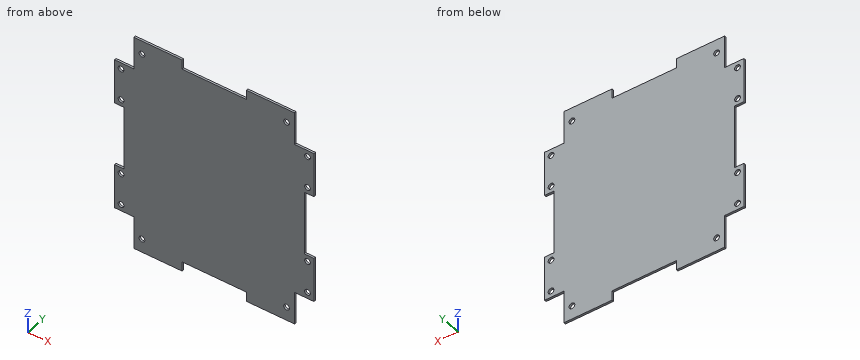
from build123d import *

# Parameters (mm, degrees)
SKETCH1_R           = 2.286
BOSS_EXTRUDE1_DEPTH = 1.5875
SKETCH2_R           = 2.286
CUT_EXTRUDE1_DEPTH  = 2.5875


with BuildPart() as part:
    # Sketch1 → Boss-Extrude1 (new body)
    with BuildSketch(Plane(origin=(0, 0, 0), x_dir=(1, 0, 0), z_dir=(0, 1, 0))):
        Polygon((-25.4, 86.995), (-63.43142, 86.995), (-63.43142, 60.96), (-78.74, 60.96), (-78.74, 25.4), (-71.12, 25.4), (-71.12, -25.4), (-78.74, -25.4), (-78.74, -60.96), (-63.43142, -60.96), (-63.43142, -86.995), (-25.4, -86.995), (-25.4, -79.375), (25.4, -79.375), (25.4, -86.995), (63.43142, -86.995), (63.43142, -60.96), (78.74, -60.96), (78.74, -25.4), (71.12, -25.4), (71.12, 25.4), (78.74, 25.4), (78.74, 60.96), (63.43142, 60.96), (63.43142, 86.995), (25.4, 86.995), (25.4, 79.375), (-25.4, 79.375), align=None)
        with Locations((-57.15, 76.2)):
            Circle(SKETCH1_R, mode=Mode.SUBTRACT)
        with Locations((57.15, 76.2)):
            Circle(SKETCH1_R, mode=Mode.SUBTRACT)
        with Locations((57.15, -76.2)):
            Circle(SKETCH1_R, mode=Mode.SUBTRACT)
        with Locations((-57.15, -76.2)):
            Circle(SKETCH1_R, mode=Mode.SUBTRACT)
    extrude(amount=BOSS_EXTRUDE1_DEPTH)

    # Sketch2 → Cut-Extrude1 (cut, through all)
    with BuildSketch(Plane(origin=(0, 1.5875, 0), x_dir=(1, 0, 0), z_dir=(0, 1, 0))):
        with Locations((-73.66, -30.48)):
            Circle(SKETCH2_R)
        with Locations((-73.66, -55.88)):
            Circle(SKETCH2_R)
        with Locations((73.66, -55.88)):
            Circle(SKETCH2_R)
        with Locations((73.66, -30.48)):
            Circle(SKETCH2_R)
        with Locations((73.66, 30.48)):
            Circle(SKETCH2_R)
        with Locations((73.66, 55.88)):
            Circle(SKETCH2_R)
        with Locations((-73.66, 55.88)):
            Circle(SKETCH2_R)
        with Locations((-73.66, 30.48)):
            Circle(SKETCH2_R)
    extrude(amount=-CUT_EXTRUDE1_DEPTH, mode=Mode.SUBTRACT)


solid = part.part
Geometry: final body of the model. Coordinates: model frame, mm. Give positions to 0.01 mm unless a question says otherwise; leave off trailing zeros. Write each loop counter-clockwise with the first axis right and the second up, starting at its lowest first coordinate (ties: lowest second). Pieces come first, ordered by that corner, then holes.
(1) Cut plane A-A, the plane x = 57.15. Return loops of the section in (y, z) (1 decimal).
(2) Cut plane B-B, the plane x = -73.66. Return loops of the section in (y, z).
(3) Ray query, line 1 (X direction, y = 0.9, z = 55.88); line 2 (Z direction, x = 57.15, y = 0.6) (3 decimals); line 3 (Z direction, x = 73.66, y = 1). Return the intervals inside material, ascending.
(4) Cut plane D-D, the plane y = 0.9. Give the number of separate pieces and of enclosed holes in the cut face, then the cut area to 3 significant figures.
(5) First-contact query: P1, Ø3.5, axis at x = -73.66, z = -30.48, coming from the -Y side; P2, Ø0.8, axis at x = -73, y = 0.5, coming from the +Z side; P3, Ø0.8, axis at y = 0.5, z = -68, coming from the +X side. Flat tips, straight axial feed; report the tip coordinate or a pass-through.
(6) Cut plane C-C, the plane z = 76.2. Return loops of the section in (x, y), then the cut area to 3 significant figures.
Values follow:
1. outline: (0, -87) - (1.6, -87) - (1.6, -78.5) - (0, -78.5) - close; (0, -73.9) - (1.6, -73.9) - (1.6, 73.9) - (0, 73.9) - close; (0, 78.5) - (1.6, 78.5) - (1.6, 87) - (0, 87) - close
2. outline: (0, -60.96) - (1.59, -60.96) - (1.59, -58.17) - (0, -58.17) - close; (0, -53.59) - (1.59, -53.59) - (1.59, -32.77) - (0, -32.77) - close; (0, -28.19) - (1.59, -28.19) - (1.59, -25.4) - (0, -25.4) - close; (0, 25.4) - (1.59, 25.4) - (1.59, 28.19) - (0, 28.19) - close; (0, 32.77) - (1.59, 32.77) - (1.59, 53.59) - (0, 53.59) - close; (0, 58.17) - (1.59, 58.17) - (1.59, 60.96) - (0, 60.96) - close
3. line 1: x = -78.74 to -75.95, -71.37 to 71.37, 75.95 to 78.74
3. line 2: z = -86.995 to -78.486, -73.914 to 73.914, 78.486 to 86.995
3. line 3: z = -60.96 to -58.17, -53.59 to -32.77, -28.19 to -25.4, 25.4 to 28.19, 32.77 to 53.59, 58.17 to 60.96
4. separate pieces: 1
4. enclosed holes: 12
4. area: 24,100 mm2
5. P1: passes through
5. P2: stops at z = 60.96
5. P3: stops at x = 63.43
6. outline: (-63.43, 0) - (-59.44, 0) - (-59.44, 1.59) - (-63.43, 1.59) - close; (-54.86, 0) - (54.86, 0) - (54.86, 1.59) - (-54.86, 1.59) - close; (59.44, 0) - (63.43, 0) - (63.43, 1.59) - (59.44, 1.59) - close
6. area: 187 mm2
